Autodesk Inventor part; units mm, degrees
ref_plane "YZ Plane" through (0, 0, 0) normal (1, 0, 0) x (0, 1, 0)
ref_plane "XZ Plane" through (0, 0, 0) normal (0, 1, 0) x (-1, 0, 0)
ref_plane "XY Plane" through (0, 0, 0) normal (0, 0, 1) x (1, 0, 0)
sketch "Sketch1" plane through (0, 0, 0) normal (0, 1, 0) x (-1, 0, 0)
  line L0 (75, -60) -> (-75, -60)
  line L1 (-75, -60) -> (-75, 60)
  line L2 (-75, 60) -> (75, 60)
  line L3 (75, 60) -> (75, -60)
  line L4 (75, -60) -> (-75, 60) construction
  line L5 (-75, -60) -> (75, 60) construction
  point P0 (0, 0)
  dimension "d0" = 120
  dimension "d1" = 150
extrude "Extrusion1" add sketch "Sketch1" along normal blind 50.5
sketch "Sketch14" plane through (0, 0, 0) normal (0, 1, 0) x (1, 0, 0)
  line L0 (-75, -60) -> (75, -60)
  line L1 (75, -60) -> (75, 60)
  line L2 (75, 60) -> (-75, 60)
  line L3 (-75, 60) -> (-75, -60)
  line L4 (0, 0) -> (0, -250) construction
  circle A0 centre (0, -250) radius 260
  circle A1 centre (0, -250) radius 291.5
  circle A2 centre (0, -250) radius 228.5
  point P0 (75, 31.6864)
  point P1 (-75, 31.6864)
  point P2 (-75, -34.1592)
  point P3 (75, -34.1592)
  dimension "d52" = 250
  dimension "d53" = 520
  dimension "d54" = 583
  dimension "d55" = 457
extrude "Extrusion13" cut sketch "Sketch14" along normal blind 45 contours L3 A0 L1 A2 | L3 A1 L1 A0 picked at (-61.8874, -8.4536) picked at (67.9829, 11.6585)
sketch "Sketch15" plane through (0, 45, 0) normal (0, -1, 0) x (1, 0, 0)
  line L0 (0, 0) -> (0, 250) construction
  circle A0 centre (0, 250) radius 260
  circle A1 centre (0, 250) radius 302.5
  circle A2 centre (0, 250) radius 217.5
  line L1 (-75, 60) -> (75, 60)
  line L2 (75, 60) -> (75, -60)
  line L3 (75, -60) -> (-75, -60)
  line L4 (-75, -60) -> (-75, 60)
  point P0 (-75, -43.055)
  point P1 (75, -43.055)
  point P2 (75, 45.8401)
  point P3 (-75, 45.8401)
  dimension "d58" = 250
  dimension "d59" = 520
  dimension "d60" = 605
  dimension "d61" = 435
extrude "Extrusion14" cut sketch "Sketch15" along normal blind 35 contours L4 A2 L2 A0 | A0 L2 A1 L4 picked at (-61.9043, 12.2496) picked at (67.9829, -15.4481)
sketch "Sketch16" plane through (0, 50.5, 0) normal (0, 1, 0) x (1, 0, 0)
  line L0 (0, 0) -> (50, 0) construction
  line L1 (0, 0) -> (-50, 0) construction
  line L2 (-50, 0) -> (-50, -25)
  line L3 (-50, -25) -> (50, -25)
  line L4 (50, -25) -> (50, 0)
  line L5 (50, 0) -> (50, 25)
  line L6 (50, 25) -> (-50, 25)
  line L7 (-50, 25) -> (-50, 0)
  dimension "d64" = 50
  dimension "d65" = 50
  dimension "d66" = 25
  dimension "d67" = 25
extrude "Extrusion15" cut sketch "Sketch16" against normal blind 3
sketch "Sketch17" plane through (0, 10, 0) normal (0, 1, 0) x (1, 0, 0)
  line L0 (0, 0) -> (-33, 0) construction
  line L1 (0, 0) -> (33, 0) construction
  line L2 (33, 0) -> (33, -35.018)
  arc A0 (75, -45.8401) -> (-75, -45.8401) centre (0, -250) ccw
  line L3 (33, 0) -> (68.018, 0) construction
  line L4 (-31.2481, 0) -> (6.0348, 0) construction
  line L5 (-33, 0) -> (-33, -35.018)
  line L6 (-33, 0) -> (2.018, 0) construction
  line L7 (-33, 0) -> (-33, 50.6946)
  arc A1 (75, 43.055) -> (-75, 43.055) centre (0, -250) ccw
  line L8 (-33, 0) -> (17.6946, 0) construction
  line L9 (33, 0) -> (33, 50.6946)
  line L10 (33, 0) -> (83.6946, 0) construction
  dimension "d70" = 33
  dimension "d71" = 33
  dimension "d72" = 90
  dimension "d74" = 90
  dimension "d75" = 90
  dimension "d76" = 90
extrude "Extrusion16" cut sketch "Sketch17" against normal blind 7
sketch "Sketch18" plane through (75, 0, -60) normal (1, 0, 0) x (0, 0, -1)
  line L0 (-94.1592, 10) -> (-105.8401, 10)
  line L1 (-105.8401, 10) -> (-105.8401, 45)
  line L2 (-105.8401, 45) -> (-16.945, 45)
  line L3 (-16.945, 45) -> (-16.945, 10)
  line L4 (-16.945, 10) -> (-28.3136, 10)
  line L5 (-28.3136, 10) -> (-28.3136, 0)
  line L6 (-28.3136, 0) -> (0, 0)
  line L7 (0, 0) -> (0, 50.5)
  line L8 (-120, 50.5) -> (0, 50.5)
  line L9 (-120, 0) -> (-120, 50.5)
  line L10 (-120, 0) -> (-94.1592, 0)
  line L11 (-94.1592, 0) -> (-94.1592, 10)
  line L12 (-60, 0) -> (-60, 50.5) construction
  line L13 (-94.1592, 10) -> (-28.3136, 10)
  line L14 (-60, 10) -> (-111, 10)
  line L15 (-111, 10) -> (-111, 45)
  line L16 (-16.945, 10) -> (-9.3054, 10)
  line L17 (-28.3136, 10) -> (-9.3054, 10)
  line L18 (-9.3054, 10) -> (-9.3054, 3)
  line L19 (-9.3054, 10) -> (-9.3054, 45)
  line L20 (-111, 45) -> (-105.8401, 45)
  line L21 (-9.3054, 45) -> (-16.945, 45)
  line L22 (-111, 45) -> (-116, 45)
  line L23 (-116, 45) -> (-116, 10)
  line L24 (-116, 10) -> (-111, 10)
  line L25 (-9.3054, 45) -> (-4.3054, 45)
  line L26 (-4.3054, 45) -> (-4.3054, 10)
  line L27 (-4.3054, 10) -> (-9.3054, 10)
  line L28 (-116, 45) -> (-116, 50.5)
  line L29 (-116, 10) -> (-116, 0)
  line L30 (-94.1592, 0) -> (-120, 0)
  line L31 (-4.3054, 45) -> (-4.3054, 50.5)
  line L32 (-4.3054, 10) -> (-4.3054, 0)
  line L33 (-111, 45) -> (-111, 50.5)
  line L34 (-9.3054, 45) -> (-9.3054, 50.5)
  line L35 (-9.3054, 10) -> (-9.3054, 0)
  line L36 (-111, 10) -> (-111, 0)
  point P0 (-9.3054, 3)
  dimension "d79" = 51
  dimension "d81" = 5
  dimension "d82" = 5
extrude "Extrusion17" cut sketch "Sketch18" against normal up to surface (150 mm away) contours L0 L1 L2 L3 L4 L13 | L24 L23 L22 L15 | L36 L10 L29 L24 | L21 L19 L16 L3 | L22 L28 L8 L33 | L29 L10 L9 L8 L28 L23 | L31 L8 L7 L6 L32 L26
sketch "Sketch19" plane through (0, 50.5, 0) normal (0, 1, 0) x (1, 0, 0)
  line L0 (75, 55.6946) -> (-75, 55.6946)
  line L1 (-75, 55.6946) -> (-75, -51)
  line L2 (-75, -51) -> (75, -51)
  line L3 (75, -51) -> (75, 55.6946)
  line L4 (50, 25) -> (50, -25)
  line L5 (50, -25) -> (-50, -25)
  line L6 (-50, -25) -> (-50, 25)
  line L7 (-50, 25) -> (50, 25)
  line L8 (50, 25) -> (50, -25) construction
  line L9 (50, -25) -> (-50, 25) construction
  line L10 (-50, -25) -> (-50, 25) construction
  line L11 (50, 25) -> (-50, -25) construction
  line L12 (50, -25) -> (-50, -25) construction
  line L13 (50, -25) -> (50, -33) construction
  line L14 (50, -33) -> (60, -33) construction
  line L15 (50, 25) -> (50, 37) construction
  line L16 (50, 37) -> (60, 37) construction
  circle A0 centre (60, -33) radius 5
  circle A1 centre (60, 37) radius 5
  line L17 (0, -51) -> (0, 55.6946) construction
  circle A2 centre (-60, -33) radius 5
  circle A3 centre (-60, 37) radius 5
  dimension "d93" = 8
  dimension "d94" = 10
  dimension "d95" = 12
  dimension "d96" = 10
  dimension "d97" = 90
  dimension "d98" = 10
  dimension "d99" = 10
extrude "Extrusion18" cut sketch "Sketch19" against normal blind 10 contours A0 | A1 | A2 | A3
properties part number "Battery Cage" material "PLA Plastic"
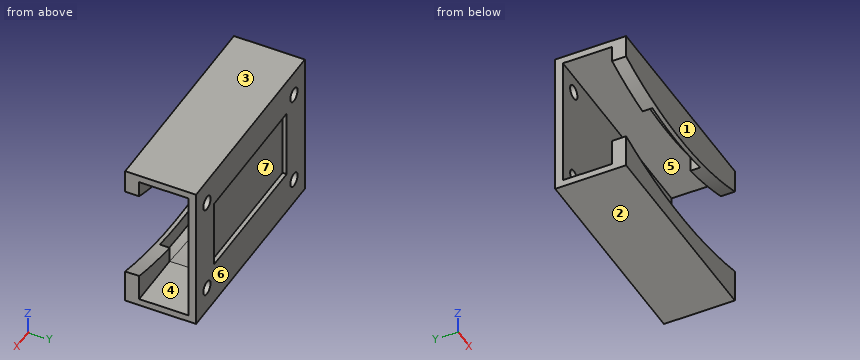
Can you work these out from the model? Positions are in its coordinate system, mm. Face numbers are marked on the shaded views. A direction names the side the tool comes from. Round coordinates to 2 decimals unless told otherwise and drop trailing zeros. Loops run counter-clockwise (first coordinate to the right, second up) from the corner with the lowest first, then second, coordinate; pieces in that order, holes last. Notation, with made-up numbers: M 55,6 L 91,6 A4 ccw 91,10 Z; hole C 6,-8.5 d3. An arc over 180 degrees is marked long. Answer as a JSON object with one key per item and string values. Group by question number.
Q1. Please list where these lines run through material, in increasing order: L1, parallel to Z at x = 60, y = 47.8; L2, parallel to X at y = 48, z = 33; L3, parallel to Y at x = -24.5, z = 44.
Q2. Will these pins go through, and if not, where does the flat tip stop? pin 1 (8 mm diameter, centred on x = 60, z = -37, fed in from +Y); pin 2 (3 mm diameter, centred on x = -28, z = -14, fed in from -Y); pin 3 (15 mm diameter, centred on x = 15, z = -8.5, fed in from +Y).
Q3. We'd pull the mould along Z, two halves only. Please class the marked faces 1, 2, 3 and 4: +Z half, -Z half, draft (parallel to the pull), parting line (faces both ways), or undercut.
Q4. On a 3-axis mill with a long thin cutter (end or side, diameter ignored), from which of +Z, -Z, +X, -X, +Y, -Y can I reach the whole of each face in a straight line? I mean the marked faces 5, 6 and 7. Say none if no direction works.
Q5. Imagine slicing it at B-B, the plane z = -37. Please give me the cut outline in (x, y).
Q6. Imagine slicing it at A-A, the plane z = 42. Please give me the cut outline in (x, y).
Q7. Imagine slicing it at C-C, the plane x = -60. Please give me the cut outline in (y, z), then the cut area to 3 significant figures.
Findings:
{
 "1": {"L1": "z = -55.69 to -42, -32 to 28, 38 to 51", "L2": "x = -75 to -65, -55 to 55, 65 to 75", "L3": "y = 0 to 10, 45 to 50.5"},
 "2": {"pin 1": "stops at y = 10", "pin 2": "stops at y = 45", "pin 3": "stops at y = 47.5"},
 "3": {"face 1": "draft", "face 2": "-Z half", "face 3": "+Z half", "face 4": "undercut"},
 "4": {"face 5": "+X, -X", "face 6": "+Z, -Z, +X, -X, +Y", "face 7": "+Y"},
 "5": {"outline": "M -75,0 L -51.02,0 L -51.02,10 L -75,10 Z; M -75,45 L -65,45 L -65,50.5 L -75,50.5 Z; M -55,45 L 55,45 L 55,50.5 L -55,50.5 Z; M 51.02,0 L 75,0 L 75,10 L 51.02,10 Z; M 65,45 L 75,45 L 75,50.5 L 65,50.5 Z"},
 "6": {"outline": "M -75,0 L 75,0 L 75,10 L -75,10 Z; M -75,45 L 75,45 L 75,50.5 L -75,50.5 Z"},
 "7": {"outline": "M 0,-55.69 L 50.5,-55.69 L 50.5,-42 L 45,-42 L 45,-50.69 L 10,-50.69 L 10,-35.26 L 0,-35.26 Z; M 0,29.52 L 10,29.52 L 10,45.84 L 45,45.84 L 45,38 L 50.5,38 L 50.5,51 L 0,51 Z; M 45,-32 L 50.5,-32 L 50.5,28 L 45,28 Z", "area": "1,250 mm2"}
}
